```python
from build123d import *

# Parameters (mm, degrees)
BOSS_EXTRUDE1_DEPTH = 4.7752
SKETCH3_W           = 4.7752
SKETCH3_H           = 4.7752
SKETCH3_W_2         = 9.292163612
SKETCH3_W_3         = 8.132236388
CUT_EXTRUDE2_DEPTH  = 6.35
SKETCH6_W           = 4.7752
SKETCH6_H           = 12.7
CUT_EXTRUDE3_DEPTH  = 6.35


with BuildPart() as part:
    # Sketch2 → Boss-Extrude1 (new body)
    with BuildSketch(Plane.XY):
        Polygon((0, 0), (38.1, 0), (38.1, 82.55), (19.05, 101.6), (0, 101.6), align=None)
    extrude(amount=BOSS_EXTRUDE1_DEPTH)

    # Sketch3 → Cut-Extrude2 (cut)
    with BuildSketch(Plane.XY.offset(4.7752)):
        with Locations((2.3876, 2.3876)):
            Rectangle(SKETCH3_W, SKETCH3_H)
        with Locations((15.771281806, 2.3876)):
            Rectangle(SKETCH3_W_2, SKETCH3_H)
        with Locations((29.258681806, 2.3876)):
            Rectangle(SKETCH3_W_3, SKETCH3_H)
    extrude(amount=-CUT_EXTRUDE2_DEPTH, mode=Mode.SUBTRACT)

    # Sketch6 → Cut-Extrude3 (cut)
    with BuildSketch(Plane.XY.offset(4.7752)):
        with Locations((2.3876, 17.4752)):
            Rectangle(SKETCH6_W, SKETCH6_H)
        with Locations((2.3876, 42.8752)):
            Rectangle(SKETCH6_W, SKETCH6_H)
        with Locations((2.3876, 68.2752)):
            Rectangle(SKETCH6_W, SKETCH6_H)
        with Locations((35.7124, 57.15)):
            Rectangle(SKETCH6_W, SKETCH6_H)
        with Locations((35.7124, 31.75)):
            Rectangle(SKETCH6_W, SKETCH6_H)
    extrude(amount=-CUT_EXTRUDE3_DEPTH, mode=Mode.SUBTRACT)


solid = part.part
```
Input: part model. Units: mm. Frame: model coordinates. A direction names the side the tool comes from. Give positions to 0.01 mm unless a question says otherwise; leave off trailing zeros. Order: outer loops, then holes, each group sorted by start corner. A loop starts at its lowest first (then second) coordinate and runs counter-clockwise, first axis right, second up.
1. Section C-C on y = 93.5. Return the cut outline in (x, z), and give its area (3 significant figures).
Derived:
outline: (0, 0) - (27.15, 0) - (27.15, 4.78) - (0, 4.78) - close
area: 130 mm2
2. Pin query (flat end, axial travel): pin 1 (1.4 mm diameter, centred on y = 1.5, z = 2.5, fed in from -X); pin 2 (2.5 mm diameter, centred on x = 36, z = 2, fed in from +Y); pin 3 (2.5 mm diameter, centred on x = 1.5, z = 2, fed in from -Y). Return the tip coordinate at first contact, or that it passes through.
Derived:
pin 1: stops at x = 4.78
pin 2: stops at y = 85.9
pin 3: stops at y = 4.78
3. Mould query, pull axis Y, two halves, no side actions, for faces 5 (the flat face through (0, 88, 2)), 6 (the flat face through (4.775, 17, 2)), 7 (the flat face through (36, 38.1, 2)), 8 (the flat face through (16, 4.775, 2)). Classes: released by +Y, released by -Y, zero draft, split by the parting line, or undercut.
Derived:
face 5: zero draft
face 6: undercut
face 7: undercut
face 8: released by -Y
4. Section A-A on x = 3.5. Return the cut outline in (y, z), and give its area (3 significant figures).
Derived:
outline: (4.78, 0) - (11.13, 0) - (11.13, 4.78) - (4.78, 4.78) - close; (23.83, 0) - (36.53, 0) - (36.53, 4.78) - (23.83, 4.78) - close; (49.23, 0) - (61.93, 0) - (61.93, 4.78) - (49.23, 4.78) - close; (74.63, 0) - (101.6, 0) - (101.6, 4.78) - (74.63, 4.78) - close
area: 280 mm2
5. Reachability of faces 1 (the flat face through (20.417, 2, 2)), 2 (the flat face through (36, 25.4, 2)), 3 (the flat face through (4.775, 43, 2)), 4 (the flat face through (2, 4.775, 2)) from +Z, -Z, +X, -X, +Y, -Y: full face, straight path, thin tool, end or side. Return the list, or none.
Derived:
face 1: +Z, -Z, -Y
face 2: +Z, -Z, +X
face 3: +Z, -Z, -X
face 4: +Z, -Z, -X, -Y
6. Section B-B on x = 24. Return the cut outline in (y, z), and give its area (3 significant figures).
Derived:
outline: (0, 0) - (96.65, 0) - (96.65, 4.78) - (0, 4.78) - close
area: 462 mm2
7. Material intervals for L1, parallel to Y at x = 3.5, z = 2.8; L2, parallel to Y at x = 34.5, z = 1.3; L3, parallel to X at y = 67, z = 0.45, sorted ascending.
Derived:
L1: y = 4.78 to 11.13, 23.83 to 36.53, 49.23 to 61.93, 74.63 to 101.6
L2: y = 0 to 25.4, 38.1 to 50.8, 63.5 to 86.15
L3: x = 4.78 to 38.1
